from build123d import *

# Parameters (mm, degrees)
F0_R     = 11.61063
F1_DEPTH = 38.1
F2_R     = 5.08
F3_SIZE  = 1.27
F5_R     = 1.777125
F6_DEPTH = 54.864


with BuildPart() as f1:
    # F0 (on Front) → F1 (new body)
    with BuildSketch(Plane.XZ):
        with BuildLine():
            Line((0, -40.706848), (0, -25.273476))
            ThreePointArc((0, -25.273476), (4.263921, 24.911194), (-8.405601, -23.834733))
            Line((-8.405601, -23.834733), (0, -40.706848))
        make_face()
        Circle(F0_R, mode=Mode.SUBTRACT)
    extrude(amount=F1_DEPTH)

    # F2
    f2_edges = [f1.edges().sort_by_distance(p)[0] for p in [
        (-11.61063, 0, 0),
        (-11.61063, -38.1, 0),
    ]]
    fillet(f2_edges, radius=F2_R)

    # F3
    f3_edges = [f1.edges().sort_by_distance(p)[0] for p in [
        (4.263921, -38.1, 24.911194),
        (0, -38.1, -32.990162),
        (4.263921, 0, 24.911194),
        (0, 0, -32.990162),
        (-4.2028, 0, -32.27079),
        (-4.2028, -38.1, -32.27079),
    ]]
    chamfer(f3_edges, length=F3_SIZE)

    # F5 (on face) → F6 (join)
    with BuildSketch(Plane.XZ.offset(38.1)):
        with Locations((-10.195103, 19.407116)):
            Circle(F5_R)
    extrude(amount=F6_DEPTH)


solid = f1.part
Source: CAD feature listing. Evaluate the final solid. Frame: model axes, mm. A direction names the side the tool comes from. Give positions to 0.01 mm unless a question says otherwise; leave off trailing zeros. Write each loop counter-clockwise with the first axis right and the second up, starting at its lowest first coordinate (ties: lowest second). Pieces come first, ordered by that corner, then holes. Notation, with made-up numbers: (-10, 1) -> (22, 1) arc R20 ccw to (22, 10) -> close; hole circle Ø7 at (6.5, 85.25). An arc over 180 degrees is marked (long way). Write item = value, one per line.
Q1. Cut plane C-C on y = -48. Return loops of the section in (x, z), then the cut area to 3 significant figures.
Here are the results:
outline = circle Ø3.55 at (-10.2, 19.41)
area = 9.92 mm²
Q2. First-contact query: pin 1 (2 mm diameter, centred on y = -13.5, z = -27, fed in from -X); pin 2 (6 mm diameter, centred on y = -16.5, z = -20.5, fed in from -X); pin 3 (14.5 mm diameter, centred on x = 7, z = -2.5, fed in from -Y). Flat tips, straight axial feed; report the tip coordinate or a pass-through.
Here are the results:
pin_1 = -7.33
pin_2 = -18.23
pin_3 = -37.69
Q3. Mould query, pull axis Z, two halves, no side actions, for faces 4 (the face through (-4.779, -37.456, -29.71)), 5 (the face through (-9, -38.1, -14.3)), 6 (the face through (11.074, -18.854, 3.488)). Classes: +Z half, -Z half, draft (parallel to the pull), parting line (faces both ways), or undercut.
Here are the results:
face_4 = -Z half
face_5 = draft
face_6 = undercut
Q4. Reachability of faces 1 (the face through (-4.779, -0.644, -29.71)), 2 (the face through (0, -19, -33)), 3 (the face through (-10.43, -65.15, 21.17)) from +Z, -Z, +X, -X, +Y, -Y: full face, straight path, thin tool, end or side. Return the list, or none.
Here are the results:
face_1 = -Z, -X, +Y
face_2 = -Z, +X, +Y, -Y
face_3 = -Y
Q5. Line query: line 1 (Y direction, x = 20.5, z = -8); line 2 (Z direction, x = 3.5, y = -36.5); line 3 (Z direction, x = 17.5, y = -33). Output: solid intervals per line, ascending. Write a range as from..to.
Here are the results:
line_1 = -38.1..0
line_2 = -25.03..-12.51, 12.51..25.03
line_3 = -18.23..18.23
Q6. Cut plane B-B on y = -25.5. Return loops of the section in (x, z).
Here are the results:
outline = (-8.41, -23.83) -> (0, -40.71) -> (0, -25.27) arc R25.27 ccw (long way) to start; hole circle Ø23.22 at (0, 0)
Q7. Cut plane A-A on z = -27. Return loops of the section in (x, y), then the cut area to 3 significant figures.
Here are the results:
outline = (-6.83, -36.83) -> (-5.41, -38.1) -> (-1.27, -38.1) -> (0, -36.83) -> (0, -1.27) -> (-1.27, 0) -> (-5.41, 0) -> (-6.83, -1.27) -> close
area = 257 mm²
